Autodesk Inventor part; units mm, degrees
ref_plane "YZ Plane" through (0, 0, 0) normal (1, 0, 0) x (0, 1, 0)
ref_plane "XZ Plane" through (0, 0, 0) normal (0, 1, 0) x (-1, 0, 0)
ref_plane "XY Plane" through (0, 0, 0) normal (0, 0, 1) x (1, 0, 0)
sketch "Sketch1" plane through (0, 0, 0) normal (0, 0, 1) x (1, 0, 0)
  line L0 (0, 0) -> (24.55, 0)
  line L1 (24.55, 0) -> (24.55, -60)
  line L2 (24.55, -60) -> (0, -60)
  line L3 (0, -60) -> (0, 0)
  dimension "d0" = 24.55
  dimension "d1" = 60
extrude "Extrusion1" add sketch "Sketch1" along normal blind 10
sketch "Sketch2" plane through (0, 0, 10) normal (0, 0, 1) x (1, 0, 0)
  line L0 (24.55, 0) -> (0, 0)
  line L1 (3, -3) -> (21.55, -3)
  line L2 (21.55, -3) -> (21.55, -57)
  line L3 (21.55, -57) -> (3, -57)
  line L4 (3, -57) -> (3, -3)
  line L5 (0, -60) -> (24.55, -60)
  line L6 (24.55, -60) -> (24.55, 0)
  line L7 (0, 0) -> (0, -60)
  dimension "d8" = 3
  dimension "d9" = 3
  dimension "d10" = 3
  dimension "d11" = 3
extrude "Extrusion2" cut sketch "Sketch2" against normal blind 8 contours L1 L2 L3 L4
sketch "Sketch3" plane through (24.55, -60, 0) normal (1, 0, 0) x (0, 0, -1)
  line L0 (-10, 44.65) -> (-2, 44.65)
  line L1 (-2, 3) -> (-2, 57)
  line L2 (-10, 13.35) -> (-2, 13.35)
  line L3 (-2, 13.35) -> (-2, 44.65)
  line L4 (-10, 13.35) -> (-10, 44.65)
  line L5 (-10, 3) -> (-10, 57)
  line L6 (0, 60) -> (-10, 60)
  line L7 (0, 0) -> (-10, 0)
  dimension "d16" = 8
  dimension "d18" = 15.35
  dimension "d19" = 13.35
extrude "Extrusion3" cut sketch "Sketch3" against normal blind 24.55
sketch "Sketch4" plane through (0, 0, 0) normal (0, 1, 0) x (1, 0, 0)
  line L0 (4.375, -10) -> (4.375, -2)
  line L1 (21.55, -2) -> (3, -2)
  line L2 (4.375, -2) -> (20.175, -2)
  line L3 (20.175, -2) -> (20.175, -10)
  line L4 (20.175, -10) -> (4.375, -10)
  line L5 (24.55, 0) -> (24.55, -10)
  point P0 (0, 0)
  dimension "d23" = 15.8
  dimension "d24" = 4.375
  dimension "d25" = 8
  dimension "d26" = 15.8
extrude "Extrusion4" cut sketch "Sketch4" against normal blind 3
properties part number "tapaArduino"
Could you check a few things on this model? Use its own coordinates, in mm. A direction names the side the tool comes from. Round coordinates to 2 decimals unless told otherwise and drop trailing zeros. Write each loop counter-clockwise with the first axis right and the second up, starting at its lowest first coordinate (ties: lowest second). Pieces come first, ordered by that corner, then holes. Notation, with made-up numbers: M 5.25,2 L 14.25,2 A28 ccw 14.25,33 Z; hole C 86.25,27 d3. An arc over 180 degrees is marked long. Write each question's results on one line, items separated by ' | '. Start each with the question number.
1. Imagine slicing it at A-A on z = 3.5. List the corners of the cut face in (x, y) for me (3 decimals).
2. Imagine slicing it at D-D on y = -18.5. List the corners of the cut face in (x, z) for me, and give its area (3 significant figures).
3. Imagine slicing it at C-C on y = -9.5. List the corners of the cut face in (x, z) for me.
4. Imagine slicing it at B-B on x = 2. List the corners of the cut face in (y, z) for me.
5. On a 3-axis mill with a long thin cutter (end or side, diameter ignored), from which of +Z, -Z, +X, -X, +Y, -Y can I reach the whole of each face in a straight line? I mean faces 4 (the face through (12, -58, 10)), 5 (the face through (4.375, -1, 6)), 6 (the face through (3, -52, 6)), 7 (the face through (2, -15.35, 6)), 8 (the face through (24.55, -29.6, 1.6)). Say none if no direction works.
6. I'm going to push a flat-ended pin straight in: pin 1 Ø12.5 at (x, y) = (12, -23.5) entering from +Z. Where does the tip first touch, or does it pass through?
7. Thinking about a two-plate mould opening in Y: for faces 1 (the face through (21, -3, 6)), 2 (the face through (0, -30.4, 1.6)), 3 (the face through (12, -60, 5)), which applies, +Y half, -Y half, draft (parallel to the pull), parting line (faces both ways), or undercut?
8. I need wall thicknesses on L1, parallel to X at y = -54, z = 6.5; L2, parallel to Y at x = 3.75, z = 3; L3, parallel to Y at x = 7.5, z = 3.25. Which ranges of each line are inside material? Lowest first, please. Write a range as from..to.
Result sheet:
1) outline: M 0,-60 L 24.55,-60 L 24.55,-46.65 L 21.55,-46.65 L 21.55,-57 L 3,-57 L 3,-46.65 L 0,-46.65 Z; M 0,-15.35 L 3,-15.35 L 3,-3 L 4.375,-3 L 4.375,0 L 0,0 Z; M 20.175,-3 L 21.55,-3 L 21.55,-15.35 L 24.55,-15.35 L 24.55,0 L 20.175,0 Z
2) outline: M 0,0 L 24.55,0 L 24.55,2 L 0,2 Z | area: 49.1 mm^2
3) outline: M 0,0 L 24.55,0 L 24.55,10 L 21.55,10 L 21.55,2 L 3,2 L 3,10 L 0,10 Z
4) outline: M -60,0 L 0,0 L 0,10 L -15.35,10 L -15.35,2 L -46.65,2 L -46.65,10 L -60,10 Z
5) face 4: +Z, +X, -X, +Y, -Y | face 5: +Z, +Y | face 6: +Z | face 7: +Z, +X, -X | face 8: +Z, -Z, +X, +Y, -Y
6) pin 1: stops at z = 2
7) face 1: undercut | face 2: draft | face 3: -Y half
8) L1: x = 0..3, 21.55..24.55 | L2: y = -60..-57, -3..0 | L3: y = -60..-57
